Part model, mm, in its own coordinate system. Face numbers are marked on the shaded views. A direction names the side the tool comes from. Coordinates: 2 decimals unless noted, no trailing zeros. Order: outer loops, then holes, each group sorted by start corner. A loop starts at its lowest first (then second) coordinate and runs counter-clockwise, first axis right, second up.
1) Cut at A-A (x = 0). List the corners of the cut face in (y, z) (3 decimals).
2) Cut at D-D (z = 390.5). List the corners of the cut face in (x, y) (3 decimals).
3) Tool access for the marked faces 1 and 2: list every direction of +Z, -Z, +X, -X, +Y, -Y with a clear straight run to the whole face (end or side of a thin tool).
4) Wall check: L1, parallel to Y at x = 0, z = 299.5 (1 decimal); L2, parallel to Z at x = 52, y = 117; L3, parallel to Y at x = 0, z = 294.5 (3 decimals). Give the ranges that are in metal, low to high.
5) Mould opens along X. For the marked faces 3, 4, 5 and 6 say: +X half, -X half, draft (parallel to the pull), parting line (faces both ways), or undercut.
6) Cut at B-B (y = -90). List the corners of the cut face in (x, z).
7) Pin check, flat tips, straight feed: pin 1 Ø6 at (x, y) = (-281, -56.5) entering from +Z; pin 2 Ø8 at (x, z) = (275.5, 362.5) entering from +Y. Stop position of each tip, or through.
8) Cut at C-C (x = 210). List the corners of the cut face in (y, z).
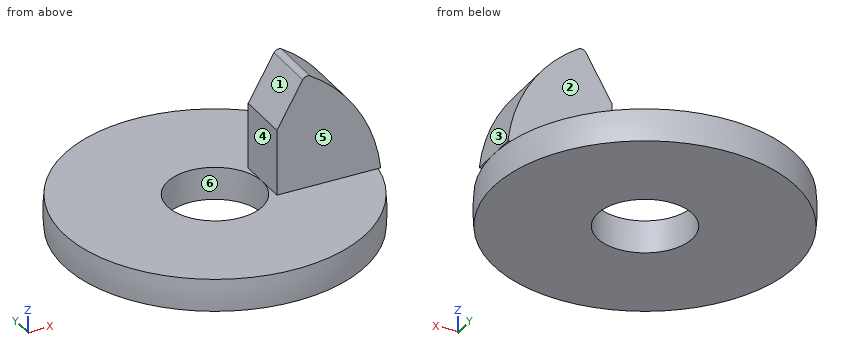
```python
from build123d import *

# Parameters (mm, degrees)
F2_DEPTH = 63.5


# Not quite as in the source:
# - a feature names something its author has since deleted; it is built from what else it names


with BuildPart() as f1:
    # F0 (on Front) → F1 (revolve)
    with BuildSketch(Plane.XZ):
        with BuildLine():
            Line((353.5530370397, 342.9), (111.125, 342.9))
            Line((111.125, 342.9), (111.125, 266.7))
            Line((111.125, 266.7), (353.5530370397, 266.7))
            ThreePointArc((353.5530370397, 266.7), (355.6, 304.8), (353.5530370397, 342.9))
        make_face()
    revolve(axis=Axis((0, 0, 509.3539357185), (0, 0, 1)))

    # F0 (on Front) → F2 (join, symmetric)
    with BuildSketch(Plane.XZ):
        with BuildLine():
            Line((111.125, 497.2741459911), (111.125, 342.9))
            Line((111.125, 342.9), (353.5530370397, 342.9))
            ThreePointArc((353.5530370397, 342.9), (301.5197040525, 493.3132039623), (189.0838855952, 605.9621560027))
            ThreePointArc((189.0838855952, 605.9621560027), (179.2716620853, 607.5323992178), (171.332367053, 601.5563647169))
            Line((171.332367053, 601.5563647169), (111.125, 497.2741459911))
        make_face()
    extrude(amount=F2_DEPTH, both=True)


solid = f1.part
```
Geometry check:
1. outline: (-353.553, 266.7) - (-111.125, 266.7) - (-111.125, 342.9) - (-353.553, 342.9) arc R355.6 ccw to start; (111.125, 266.7) - (353.553, 266.7) arc R355.6 ccw to (353.553, 342.9) - (111.125, 342.9) - close
2. outline: (111.125, -63.5) - (345.119, -63.5) - (345.119, 63.5) - (111.125, 63.5) - close
3. face 1: +Z, -X, +Y, -Y
3. face 2: +Z, +X, -X, +Y
4. L1: y = -355.6 to -111.1, 111.1 to 355.6
4. L2: z = 266.7 to 342.9
4. L3: y = -355.451 to -111.125, 111.125 to 355.451
5. face 3: +X half
5. face 4: -X half
5. face 5: draft
5. face 6: undercut
6. outline: (-341.91, 266.7) - (-65.18, 266.7) - (-65.18, 342.9) - (-341.91, 342.9) arc R344.02 ccw to start; (65.18, 266.7) - (341.91, 266.7) arc R344.02 ccw to (341.91, 342.9) - (65.18, 342.9) - close
7. pin 1: stops at z = 342.9
7. pin 2: stops at y = 63.5
8. outline: (-284.43, 266.7) - (284.43, 266.7) arc R286.97 ccw to (284.43, 342.9) - (63.5, 342.9) - (63.5, 591.77) - (-63.5, 591.77) - (-63.5, 342.9) - (-284.43, 342.9) arc R286.97 ccw to start
